Check sheet for the modelled part. Datum: model origin and axes. Units: mm. Face numbers are marked on the shaded views. A direction names the side the tool comes from. Coordinates: 2 decimals unless noted, no trailing zeros. Loops run counter-clockwise (first coordinate to the right, second up) from the corner with the lowest first, then second, coordinate; pieces in that order, holes last. Notation, with made-up numbers: M -13.75,67 L 10.25,67 A21 cw 10.25,75 Z; hole C 25,77.5 d8. An arc over 180 degrees is marked long. Write each question's results on one line, items separated by ' | '. Start each with the question number.
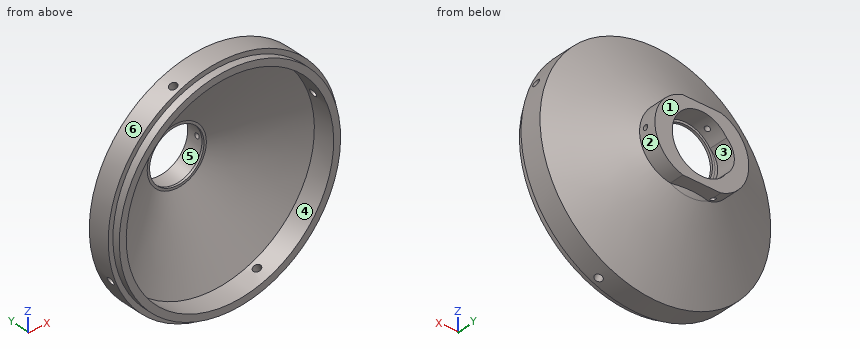
from build123d import *

# Parameters (mm, degrees)
SKETCH12_R          = 1.6425
CUT_EXTRUDE6_DEPTH  = 65.936179354
CUT_EXTRUDE7_REACH  = 38.04
SKETCH13_W          = 16.370705544
SKETCH13_H          = 2
BOSS_EXTRUDE1_REACH = 38.04
SKETCH14_R          = 12.75
CUT_EXTRUDE8_DEPTH  = 8.323317
SKETCH16_R          = 1.095
CUT_EXTRUDE9_DEPTH  = 50.7000001
CIRPATTERN2_COUNT   = 3
CIRPATTERN3_COUNT   = 4


with BuildPart() as part:
    # Sketch2 → Revolve1 (revolve)
    with BuildSketch(Plane.XY, mode=Mode.PRIVATE) as revolve1_sk:
        Polygon((49.7, 12.7), (49.7, 3.2004), (47.675, 3.2004), (47.675, 0), (44.7, 0), (44.7, 9.696683305), (12.75, 26.696683305), (11.73, 26.696683305), (11.73, 27.716683305), (12.75, 27.716683305), (12.75, 36.04), (17.75, 36.04), (17.75, 29.7), align=None)
    revolve(revolve1_sk.sketch.rotate(Axis((0, 0, 0), (0, 1, 0)), 90), axis=Axis((0, 0, 0), (0, 1, 0)))  # turned: the seam where the file's is

    # Sketch12 → Cut-Extrude6 (cut, through all)
    with BuildSketch(Plane(origin=(0, 0, 0), x_dir=(0.923879533, 0, 0.382683432), z_dir=(-0.382683432, 0, 0.923879533))):
        with Locations((0, 6.35)):
            Circle(SKETCH12_R)
    cut_extrude6 = extrude(amount=-CUT_EXTRUDE6_DEPTH, mode=Mode.SUBTRACT)

    # Cut-Extrude7: up to this cone (the profile starts outside it)
    cut_extrude7_end = Plane(origin=(0, 36.04, 0), z_dir=(0, -1, 0)).offset(-3.104443444) * Cone(1.879e-06, 89.232542042, 47.478972856, align=(Align.CENTER, Align.CENTER, Align.MIN), mode=Mode.PRIVATE)
    # Sketch13 → Cut-Extrude7 (cut, up to the surface)
    with BuildSketch(Plane(origin=(0, 36.04, 0), x_dir=(1, 0, 0), z_dir=(0, 1, 0)), mode=Mode.PRIVATE) as cut_extrude7_sk1:
        with Locations((0, 16.75)):
            Rectangle(SKETCH13_W, SKETCH13_H)
    cut_extrude7_tool1 = extrude(cut_extrude7_sk1.sketch, amount=-CUT_EXTRUDE7_REACH, mode=Mode.PRIVATE) - cut_extrude7_end
    add(cut_extrude7_tool1.solids().sort_by_distance((0, 36.04, -16.75))[0], mode=Mode.SUBTRACT)
    # Sketch13 → Cut-Extrude7 (cut, up to the surface)
    with BuildSketch(Plane(origin=(0, 36.04, 0), x_dir=(1, 0, 0), z_dir=(0, 1, 0)), mode=Mode.PRIVATE) as cut_extrude7_sk2:
        with Locations((0, -16.75)):
            Rectangle(SKETCH13_W, SKETCH13_H)
    cut_extrude7_tool2 = extrude(cut_extrude7_sk2.sketch, amount=-CUT_EXTRUDE7_REACH, mode=Mode.PRIVATE) - cut_extrude7_end
    add(cut_extrude7_tool2.solids().sort_by_distance((0, 36.04, 16.75))[0], mode=Mode.SUBTRACT)

    # Boss-Extrude1: up to this cone (the profile starts outside it)
    boss_extrude1_end = Plane(origin=(0, 36.04, 0), z_dir=(0, -1, 0)).offset(-3.104443444) * Cone(1.879e-06, 89.232542042, 47.478972856, align=(Align.CENTER, Align.CENTER, Align.MIN), mode=Mode.PRIVATE)
    # Sketch14 → Boss-Extrude1 (add, up to the surface)
    with BuildSketch(Plane(origin=(0, 36.04, 0), x_dir=(1, 0, 0), z_dir=(0, 1, 0)), mode=Mode.PRIVATE) as boss_extrude1_sk1:
        with BuildLine():
            Line((-8.185352772, 15.75), (8.185352772, 15.75))
            ThreePointArc((8.185352772, 15.75), (20.25, 0), (8.185352772, -15.75))
            Line((8.185352772, -15.75), (-8.185352772, -15.75))
            ThreePointArc((-8.185352772, -15.75), (-20.25, 0), (-8.185352772, 15.75))
        make_face()
        with Locations(Location((0, 0, 0), (0, 0, 90))):  # turned: the seam where the file's is
            Circle(SKETCH14_R, mode=Mode.SUBTRACT)
    boss_extrude1_tool1 = extrude(boss_extrude1_sk1.sketch, amount=-BOSS_EXTRUDE1_REACH, mode=Mode.PRIVATE) - boss_extrude1_end
    add(boss_extrude1_tool1.solids().sort_by_distance((0, 36.04, 15.236921))[0])

    # Sketch15 → Cut-Extrude8 (cut)
    with BuildSketch(Plane(origin=(0, 36.04, 0), x_dir=(1, 0, 0), z_dir=(0, 1, 0))):
        with BuildLine():
            ThreePointArc((-10.656570743, 7), (-13.999716493, 0), (-10.656570743, -7))
            ThreePointArc((-10.656570743, -7), (-12.75, 0), (-10.656570743, 7))
        make_face()
    extrude(amount=-CUT_EXTRUDE8_DEPTH, mode=Mode.SUBTRACT)

    # Sketch16 → Cut-Extrude9 (cut, through all)
    with BuildSketch(Plane(origin=(0, 0, 0), x_dir=(0, 0, -1), z_dir=(1, 0, 0))):
        with Locations(Location((0, 31.368341653, 0), (0, 0, 180))):  # turned: the seam where the file's is
            Circle(SKETCH16_R)
    cut_extrude9 = extrude(amount=CUT_EXTRUDE9_DEPTH, mode=Mode.SUBTRACT)

    # CirPattern2: Cut-Extrude9 ×3 about axis
    cirpattern2_axis = Axis((0, 13.335, 0), (0, -1, 0))
    for i in range(1, CIRPATTERN2_COUNT):
        add(cut_extrude9.rotate(cirpattern2_axis, i * 360 / CIRPATTERN2_COUNT), mode=Mode.SUBTRACT)

    # CirPattern3: Cut-Extrude6 ×4 about axis
    cirpattern3_axis = Axis((0, 13.335, 0), (0, -1, 0))
    for i in range(1, CIRPATTERN3_COUNT):
        add(cut_extrude6.rotate(cirpattern3_axis, i * 360 / CIRPATTERN3_COUNT), mode=Mode.SUBTRACT)


solid = part.part
1) Set-up check for the marked faces 4, 5 and 6: record each of +Z, -Z, +X, -X, +Y, -Y from which the full face is reachable in a straight line by a thin tool's end or side.
2) Thickness scan on probe 1 along X at (y, z) = (6.25, 0); probe 2 along X at (y, z) = (4, 31.5); probe 3 along Y at (x, z) = (15, 0). Record the ranges inside material, lowest first.
3) Section check A-A (y = 18). Enter the section's corners in (x, z).
4) Gauge pin test, flat ends, axial feed: P1, Ø3, axis at x = -0.5, y = 32.5, coming from the +Z side; P2, Ø1, axis at x = -12.5, z = 0, coming from the +Y side; P3, Ø1.9, axis at x = -1.5, y = 32.5, coming from the -Z side. Record the tip position at first contact, or that the pin passes through.
5) Release check for a two-part mould opening along X. For the marked faces 1, 2 and 3 record: +X half, -X half, draft (parallel to the pull), parting line (faces both ways), or undercut.
Return value:
1) face 4: -Y | face 5: +Y | face 6: +Y, -Y
2) probe 1: x = -49.7 to -44.7, 44.7 to 49.7 | probe 2: x = -38.44 to -31.71, 31.71 to 38.44 | probe 3: y = 25.5 to 30.27, 32.46 to 36.04
3) outline: C 0,0 d79.48; hole C 0,0 d58.19
4) P1: stops at z = 15.75 | P2: stops at y = 27.72 | P3: stops at z = -15.75
5) face 1: draft | face 2: +X half | face 3: undercut
